Geometry check sheet. Reference: the model listing, model coordinates, mm. Coordinates: 2 decimals unless noted, no trailing zeros. Order: outer loops, then holes, each group sorted by start corner. A loop starts at its lowest first (then second) coordinate and runs counter-clockwise, first axis right, second up. Notation, with made-up numbers: (27, 10) - (47, 10) arc R32 cw to (47, 37) - close; hole circle Ø3 at (46.5, 43). An arc over 180 degrees is marked (long way). Put each result on its own line as item: value.
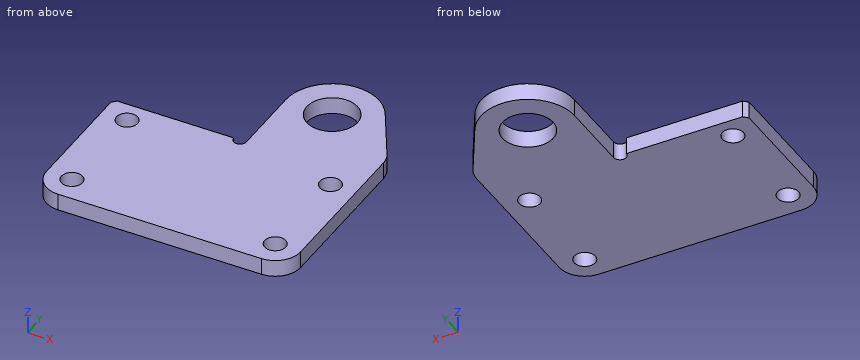
Autodesk Inventor part; units mm, degrees
ref_plane "YZ Plane" through (0, 0, 0) normal (1, 0, 0) x (0, 1, 0)
ref_plane "XZ Plane" through (0, 0, 0) normal (0, 1, 0) x (-1, 0, 0)
ref_plane "XY Plane" through (0, 0, 0) normal (0, 0, 1) x (1, 0, 0)
sketch "スケッチ1" plane through (0, 0, 0) normal (0, 0, 1) x (1, 0, 0)
  line L0 (54.882, 0) -> (12, 60) construction
  line L1 (54.882, 0) -> (70, -21.1529)
  line L2 (70, -21.1529) -> (35, -33.1249)
  line L3 (0, 0) -> (0, 100.7114)
  line L4 (0, 0) -> (54.882, 0) construction
  arc A0 (24.927, 26.5822) -> (24.2651, 18.1082) centre (58.2269, 19.7183) ccw construction
  arc A1 (17.0917, 28.1972) -> (16.274, 17.7294) centre (58.2269, 19.7183) ccw construction
  arc A2 (16.274, 17.7294) -> (24.2651, 18.1082) centre (20.2695, 17.9188) ccw construction
  line L5 (20.2695, 17.9188) -> (58.2269, 19.7183) construction
  line L6 (58.2269, 19.7183) -> (20.6135, 25.1248)
  arc A3 (20.6135, 25.1248) -> (20.2695, 17.9188) centre (58.2269, 19.7183) ccw construction
  line L7 (20.2695, 17.9188) -> (68.8874, -17.2423) construction
  line L8 (68.8874, -17.2423) -> (71.9395, 19.6224) construction
  line L9 (20.6135, 25.1248) -> (35, -33.1249)
  line L10 (20.6135, 25.1248) -> (12, 60) construction
  line L11 (20.6135, 25.1248) -> (54.882, 0) construction
  arc A4 (57.1481, -25.9011) -> (71.9395, 19.6224) centre (54.882, 0) ccw
  line L12 (35, -33.1249) -> (70, -33.1249) construction
  line L13 (70, -33.1249) -> (70, -21.1529) construction
  line L14 (27.4112, -33.1249) -> (45, -293.1249) construction
  line L15 (54.882, 0) -> (53.4072, -2.6124)
  line L16 (54.882, 0) -> (52.2839, -1.5) construction
  arc A5 (52.2839, -1.5) -> (57.7658, -0.8269) centre (54.882, 0) ccw construction
  line L17 (54.882, 0) -> (52.8265, -2.1851) construction
  line L18 (54.882, 0) -> (53.5434, -2.6848) construction
  line L19 (54.882, 0) -> (54.374, -2.9567) construction
  line L20 (54.882, 0) -> (55.2476, -2.9776) construction
  line L21 (54.882, 0) -> (56.0902, -2.7459) construction
  line L22 (54.882, 0) -> (56.8303, -2.2812) construction
  line L23 (54.882, 0) -> (57.4051, -1.6229) construction
  line L24 (54.882, 0) -> (57.7658, -0.8269) construction
  line L25 (58.2269, 19.7183) -> (53.4072, -2.6124)
  line L26 (52.2839, -1.5) -> (58.2269, 19.7183) construction
  line L27 (58.2269, 19.7183) -> (57.7658, -0.8269) construction
  line L28 (55.5792, -7.9696) -> (57.1481, -25.9011) construction
  line L29 (57.8465, -7.4305) -> (64.5165, -24.149) construction
  line L30 (59.8621, -6.2609) -> (71.0674, -20.3478) construction
  line L31 (61.4552, -4.56) -> (76.2448, -14.8199) construction
  line L32 (62.4905, -2.4721) -> (79.6095, -8.0344) construction
  line L33 (62.8801, -0.1745) -> (80.8758, -0.5672) construction
  line L34 (62.591, 2.1379) -> (79.9364, 6.9482) construction
  line L35 (61.6478, 4.2689) -> (76.8709, 13.874) construction
  line L36 (60.1305, 6.0377) -> (71.9395, 19.6224) construction
  arc A6 (55.5792, -7.9696) -> (60.1305, 6.0377) centre (54.882, 0) ccw construction
  line L37 (21.0093, 27.3897) -> (58.2269, 19.7183) construction
  arc A7 (21.0093, 27.3897) -> (20.6135, 25.1248) centre (58.2269, 19.7183) ccw construction
  arc A8 (24.927, 26.5822) -> (17.0917, 28.1972) centre (21.0093, 27.3897) ccw construction
  line L38 (52.8265, -2.1851) -> (58.2269, 19.7183) construction
  line L39 (58.2269, 19.7183) -> (20.7871, 26.2192) construction
  line L40 (20.5792, 24.8807) -> (58.2269, 19.7183) construction
  line L41 (53.5434, -2.6848) -> (58.2269, 19.7183) construction
  line L42 (21.0093, 27.3897) -> (20.7706, -32.6098) construction
  line L43 (20.7706, -32.6098) -> (57.1481, -25.9011) construction
  line L44 (20.7871, 26.2192) -> (28.6655, -33.2613) construction
  line L45 (28.6655, -33.2613) -> (64.5165, -24.149) construction
  line L46 (35, -33.1249) -> (45, -293.1249)
  line L47 (70, -21.1529) -> (45, -293.1249)
  line L48 (28.6655, -33.2613) -> (17.6783, -293.2214) construction
  line L49 (17.6783, -293.2214) -> (64.5165, -24.149) construction
  line L50 (57.1481, -25.9011) -> (-7.4742, -291.2645) construction
  line L51 (-7.4742, -291.2645) -> (20.7706, -32.6098) construction
  line L52 (58.2269, 19.7183) -> (20.4111, 23.4553) construction
  line L53 (58.2269, 19.7183) -> (20.2969, 22.0239) construction
  line L54 (58.2269, 19.7183) -> (20.2388, 20.6688) construction
  line L55 (58.2269, 19.7183) -> (20.2277, 19.4745) construction
  line L56 (58.2269, 19.7183) -> (20.2456, 18.5281) construction
  line L57 (58.2269, 19.7183) -> (54.374, -2.9567) construction
  line L58 (58.2269, 19.7183) -> (55.2476, -2.9776) construction
  line L59 (58.2269, 19.7183) -> (56.0902, -2.7459) construction
  line L60 (58.2269, 19.7183) -> (56.8303, -2.2812) construction
  line L61 (58.2269, 19.7183) -> (57.4051, -1.6229) construction
  line L62 (20.5792, 24.8807) -> (36.3145, -33.0192) construction
  line L63 (36.3145, -33.0192) -> (71.0674, -20.3478) construction
  line L64 (76.2448, -14.8199) -> (43.4556, -31.9429) construction
  line L65 (43.4556, -31.9429) -> (20.4111, 23.4553) construction
  line L66 (20.2969, 22.0239) -> (49.9482, -30.1374) construction
  line L67 (49.9482, -30.1374) -> (79.6095, -8.0344) construction
  line L68 (80.8758, -0.5672) -> (55.7371, -27.7034) construction
  line L69 (55.7371, -27.7034) -> (20.2388, 20.6688) construction
  line L70 (20.2277, 19.4745) -> (60.8132, -24.7162) construction
  line L71 (60.8132, -24.7162) -> (79.9364, 6.9482) construction
  line L72 (76.8709, 13.874) -> (65.1878, -21.2235) construction
  line L73 (65.1878, -21.2235) -> (20.2456, 18.5281) construction
  line L74 (36.3145, -33.0192) -> (51.5259, -292.7664) construction
  line L75 (71.9395, 19.6224) -> (311.1178, -112.2394) construction
  line L76 (311.1178, -112.2394) -> (68.8874, -17.2423) construction
  line L77 (76.8709, 13.874) -> (278.0839, -170.8071) construction
  line L78 (278.0839, -170.8071) -> (65.1878, -21.2235) construction
  line L79 (60.8132, -24.7162) -> (235.5555, -217.4988) construction
  line L80 (235.5555, -217.4988) -> (79.9364, 6.9482) construction
  line L81 (80.8758, -0.5672) -> (187.8232, -251.8758) construction
  line L82 (187.8232, -251.8758) -> (55.7371, -27.7034) construction
  line L83 (49.9482, -30.1374) -> (138.9893, -274.6199) construction
  line L84 (138.9893, -274.6199) -> (79.6095, -8.0344) construction
  line L85 (76.2448, -14.8199) -> (92.626, -287.4468) construction
  line L86 (92.626, -287.4468) -> (43.4556, -31.9429) construction
  line L87 (51.5259, -292.7664) -> (71.0674, -20.3478) construction
  spline S0 degree 4 poles (-7.4742, -291.2645) (-12.2705, -294.3182) (60.154, -292.0463) (27.8526, -295.3281) (110.0905, -286.5066) (139.1565, -274.7713) (216.3886, -242.7571) (259.5293, -197.6399) (297.4502, -150.2821) (311.1178, -112.2394) knots 0 0 0 0 0 0.20634 0.298589 0.40005 0.523805 0.654143 1 1 1 1 1 construction
  spline S1 degree 4 poles (20.7706, -32.6098) (25.5837, -33.2782) (32.3307, -33.6056) (40.6453, -32.8812) (49.7904, -30.3738) (57.6947, -27.0887) (63.1804, -23.3839) (66.7313, -19.9462) (68.8874, -17.2423) knots 0 0 0 0 0 0.335801 0.464563 0.589185 0.709887 1 1 1 1 1
  circle A9 centre (58.2269, 19.7183) radius 4 construction
  line L88 (0, 0) -> (0, -360.4465)
  point P0 (54.882, 0)
  point P1 (54.882, 0)
  point P2 (54.882, 0)
  point P3 (54.882, 0)
  point P4 (54.882, 0)
  point P5 (54.882, 0)
  point P6 (54.882, 0)
  point P7 (54.882, 0)
  dimension "d5" = 60
  dimension "d66" = 26
  dimension "d67" = 35
  dimension "d74" = 65
  dimension "d76" = 3
  dimension "d80" = 134
  dimension "d82" = 20
  dimension "d85" = 134
  dimension "d87" = 65
  dimension "d88" = 60
  dimension "d89" = 86
  dimension "d90" = 86
  dimension "d91" = 86
  dimension "d92" = 4
  dimension "d93" = 86
  dimension "d94" = 86
  dimension "d95" = 95
  dimension "d96" = 86
  dimension "d97" = 86
  dimension "d98" = 86
  dimension "d99" = 86
  dimension "d100" = 86
  dimension "d101" = 8
  dimension "d102" = 12
  dimension "d104" = 74.818
  dimension "d105" = 8
  dimension "d106" = 75.286
  dimension "d111" = 11.972
  dimension "d113" = 70
  dimension "d114" = 38
  dimension "d116" = 90
  dimension "d117" = 260
sketch "スケッチ2" plane through (0, 0, 0) normal (0, 0, 1) x (1, 0, 0)
  arc A0 (62.99, 22.4683) -> (52.7269, 19.7183) centre (58.2269, 19.7183) ccw
  line L0 (40, 8.7) -> (64, 8.7) construction
  line L1 (64, 8.7) -> (64, -3.3) construction
  line L2 (64, -3.3) -> (40, -3.3) construction
  line L3 (40, -3.3) -> (40, 8.7) construction
  line L4 (36, 10.1673) -> (36, -48.9437) construction
  line L5 (67, 14.719) -> (67, -3.3)
  line L6 (64, -6.3) -> (40, -6.3)
  line L7 (37, -3.3) -> (37, 10.7)
  arc A1 (37, -3.3) -> (40, -6.3) centre (40, -3.3) ccw
  arc A2 (64, -6.3) -> (67, -3.3) centre (64, -3.3) ccw
  line L8 (0, 0) -> (0, -59.5537) construction
  line L9 (10.6628, 2.7) -> (66.9205, 2.7) construction
  line L10 (66.5981, 16.219) -> (62.99, 22.4683)
  arc A3 (67, 14.719) -> (66.5981, 16.219) centre (64, 14.719) ccw
  line L11 (37.5, 11.2) -> (51.2269, 11.2)
  line L12 (52.7269, 19.7183) -> (52.7269, 11.2)
  arc A4 (51.2269, 11.2) -> (52.7269, 11.2) centre (51.9769, 11.2) ccw
  line L13 (37, 10.7) -> (37.5, 11.2)
  point P0 (67, 15.5229)
  point P1 (36.9922, 11.2)
  point P2 (37, 11.2)
  dimension "d16" = 24
  dimension "d17" = 4
  dimension "d18" = 12
  dimension "d20" = 72
  dimension "d23" = 5.5
  dimension "d108" = 3
  dimension "d109" = 30
  dimension "d118" = 2.7
  dimension "d119" = 3
  dimension "d120" = 0.75
  dimension "d121" = 0.5
  dimension "d122" = 0.5
  dimension "d124" = 8.5
extrude "押し出し1" add sketch "スケッチ2" along normal blind 2
hole "穴1" at (58.2269, 19.7183, 0) direction (0, 0, 1) diameter 6 end through all
hole "穴2" at (64, 8.7, 0) at (40, 8.7, 0) at (40, -3.3, 0) at (64, -3.3, 0) direction (0, 0, 1) diameter 2.5 end through all
equation "\"input_link_length\" = 26"
equation "\"input_link_formed_angle\" = 65deg"
equation "\"support_formed_angle\" = 86deg"
equation "\"input_slider_radius\" = 3"
equation "\"driver_rotation_range\" = 134deg"
equation "\"virtual_mass_point_x\" = 12"
equation "\"driver_min_angle\" = 95deg"
equation "\"coupler_x\" = 35"
equation "\"support_link_length\" = 38"
properties part number "COXA_YAW_SERVO_BASE"
Q1. Section check A-A on y = 8.7. Record the boundary of the cut face in (x, z).
Answer block:
outline: (37, 0) - (38.75, 0) - (38.75, 2) - (37, 2) - close; (41.25, 0) - (62.75, 0) - (62.75, 2) - (41.25, 2) - close; (65.25, 0) - (67, 0) - (67, 2) - (65.25, 2) - close
Q2. Thickness scan on L1, parallel to X at y = -3.3, z = 1; L2, parallel to Y at x = 40, z = 1.25; L3, parallel to Y at x = 63.5, z = 1.7. Record the ranges inside material, lowest first. Write a range as [from, to].
Answer block:
L1: x = [37, 38.75], [41.25, 62.75], [65.25, 67]
L2: y = [-6.3, -4.55], [-2.05, 7.45], [9.95, 11.2]
L3: y = [-6.3, -4.45], [-2.15, 7.55], [9.85, 21.58]
Q3. Section check B-B on x = 60.25. Record the boundary of the cut face in (y, z), then the cut area to 3 significant figures.
Answer block:
outline: (-6.3, 0) - (17.5, 0) - (17.5, 2) - (-6.3, 2) - close; (21.93, 0) - (24.83, 0) - (24.83, 2) - (21.93, 2) - close
area: 53.4 mm^2
Q4. Depth check by flat-ended pin: pin 1 Ø4 at (x, y) = (59, 18.5) entering from +Z; pin 2 Ø1 at (y, z) = (19.5, 1) entering from +X; pin 3 Ø2 at (x, y) = (64, -3.3) entering from -Z; pin 4 Ø0.6 at (y, z) = (14, 1) entering from -X. Enter the tip coordinate at first touch or a pass-through.
Answer block:
pin 1: stops at z = 2
pin 2: stops at x = 64.99
pin 3: passes through
pin 4: stops at x = 52.73
Q5. Section check C-C on z = 1.6. Record the boundary of the cut face in (x, y).
Answer block:
outline: (37, -3.3) arc R3 ccw to (40, -6.3) - (64, -6.3) arc R3 ccw to (67, -3.3) - (67, 14.72) arc R3 ccw to (66.6, 16.22) - (62.99, 22.47) arc R5.5 ccw to (52.73, 19.72) - (52.73, 11.2) arc R0.75 cw to (51.23, 11.2) - (37.5, 11.2) - (37, 10.7) - close; hole circle Ø2.5 at (40, -3.3); hole circle Ø2.5 at (40, 8.7); hole circle Ø6 at (58.23, 19.72); hole circle Ø2.5 at (64, -3.3); hole circle Ø2.5 at (64, 8.7)
Q6. Section check D-D on y = 20.5. Record the boundary of the cut face in (x, z).
Answer block:
outline: (52.78, 0) - (55.33, 0) - (55.33, 2) - (52.78, 2) - close; (61.12, 0) - (64.13, 0) - (64.13, 2) - (61.12, 2) - close
